CAD build for the part. Positions are in the model's coordinates, mm. Round coordinates to 2 decimals unless told otherwise and drop trailing zeros. Order: outer loops, then holes, each group sorted by start corner. A loop starts at its lowest first (then second) coordinate and runs counter-clockwise, first axis right, second up. Notation, with made-up numbers: M 36,78 L 46,78 A14 ccw 46,84 Z; hole C 84.5,38 d9. An arc over 180 degrees is marked long. Answer as CSV lines item,"result". Start each with the question number.
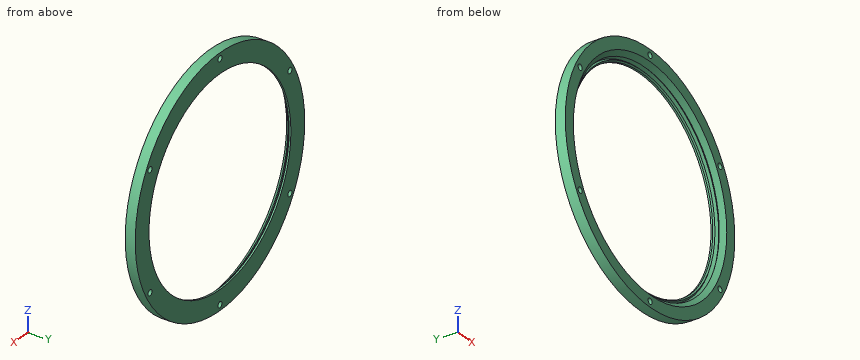
Autodesk Inventor part; units mm, degrees
ref_plane "YZ Plane" through (0, 0, 0) normal (1, 0, 0) x (0, 1, 0)
ref_plane "XZ Plane" through (0, 0, 0) normal (0, 1, 0) x (-1, 0, 0)
ref_plane "XY Plane" through (0, 0, 0) normal (0, 0, 1) x (1, 0, 0)
sketch "Sketch1" plane through (0, 0, 0) normal (0, 0, 1) x (1, 0, 0)
  line L0 (0, -12.446) -> (0, 12.446)
  line L1 (-129.54, 0) -> (21.59, 0) construction
  line L2 (-107.95, 8.89) -> (-107.95, 0)
  line L3 (-107.95, 8.89) -> (-90.3815, 8.89)
  line L4 (-90.3815, 8.89) -> (-90.3815, 7.3025)
  line L5 (-90.3815, 7.3025) -> (-91.504, 6.18)
  line L6 (-91.504, 6.18) -> (-92.9409, 7.6168)
  line L7 (-92.9409, 7.6168) -> (-95.186, 5.3717)
  line L8 (-95.186, 5.3717) -> (-93.7491, 3.9349)
  line L9 (-93.7491, 3.9349) -> (-97.684, 0)
  line L10 (-97.176, 0) -> (-88.9855, 8.1905) construction
  line L11 (-94.0634, 6.4943) -> (-92.3726, 4.8034) construction
  circle A0 centre (-93.218, 5.6489) radius 1.3081 construction
  line L12 (-107.95, -8.89) -> (-90.3815, -8.89) construction
  line L13 (-90.3815, -8.89) -> (-90.3815, -7.3025) construction
  line L14 (-90.3815, -7.3025) -> (-91.504, -6.18) construction
  line L15 (-91.504, -6.18) -> (-92.9409, -7.6168) construction
  line L16 (-92.9409, -7.6168) -> (-95.186, -5.3717) construction
  line L17 (-95.186, -5.3717) -> (-93.7491, -3.9349) construction
  line L18 (-93.7491, -3.9349) -> (-97.684, 0) construction
  line L19 (-107.95, 0) -> (-97.684, 0)
  line L20 (-107.95, 0) -> (-107.95, -8.89) construction
  point P0 (0, 0)
  dimension "d24" = 1.5875
  dimension "d25" = 2.032
  dimension "d26" = 45
  dimension "d27" = 0.508
  dimension "d28" = 3.175
  dimension "d29" = 2.6162
  dimension "d30" = 186.436
  dimension "d31" = 215.9
  dimension "d32" = 17.78
  dimension "d33" = 1.5875
revolve "Revolution1" add sketch "Sketch1" angle 360 about axis through (0, -10, 0) along (0, 1, 0)
sketch "Sketch2" plane through (0, 8.89, 0) normal (0, 1, 0) x (1, 0, 0)
  point P0 (0, 0)
  point P1 (0, 102.87)
  point P2 (-89.088, 51.435)
  point P3 (-89.088, -51.435)
  point P4 (0, -102.87)
  point P5 (89.088, -51.435)
  point P6 (89.088, 51.435)
  dimension "d36" = 102.87
  dimension "d39" = 360
hole "Hole1" at (0, 8.89, -102.87) at (-89.088, 8.89, -51.435) at (-89.088, 8.89, 51.435) at (0, 8.89, 102.87) at (89.088, 8.89, 51.435) at (89.088, 8.89, -51.435) direction (0, -1, 0) diameter 5.1054 end through all
properties part number "3DPRINT,OUTER-V" material "Nylon 6/6"
Q1. Band-saw the part on B-B, the plane z = 0. Write the cut outline in (x, y).
Q2. Drop flat-ended pins along their axis: P1, Ø1, axis at y = 5.5, z = -40.5, coming from the +X side; P2, Ø1, axis at y = 5, z = 79, coming from the -X side; P3, Ø6, axis at x = -89.088, z = 51.435, coming from the -Y side; P4, Ø2, axis at x = 19.5, y = 6.5, coming from the +Z side. Give the stop position or say it passes through.
Q3. Band-saw the part on D-D, the plane z = -102.87. Write the cut outline in (x, y).
Q4. Probe line 1 along Z through (x, y) = (2, 5); line 2 along Z through (x, y) = (6.5, 6.5); line 3 along X through (y, z) = (6.75, -71). List the from-to ranges inside material, lowest first. Write a range as from..to.
Q5. Band-saw the part on A-A, the plane x = 0. Write the cut outline in (y, z), then the cut area to 3 significant figures.
Q6. Band-saw the part on C-C, the plane y = 2.5. Write the cut outline in (x, z) (3 decimals).
Answer:
1,outline,"M -107.95,0 L -97.68,0 L -93.75,3.93 L -95.19,5.37 L -92.94,7.62 L -91.5,6.18 L -90.38,7.3 L -90.38,8.89 L -107.95,8.89 Z; M 90.38,7.3 L 91.5,6.18 L 92.94,7.62 L 95.19,5.37 L 93.75,3.93 L 97.68,0 L 107.95,0 L 107.95,8.89 L 90.38,8.89 Z"
2,P1,"stops at x = 100.27"
2,P2,"stops at x = -74.1"
2,P3,"stops at y = 0"
2,P4,"stops at z = 106.35"
3,outline,"M -32.73,0 L -2.55,0 L -2.55,8.89 L -32.73,8.89 Z; M 2.55,0 L 32.73,0 L 32.73,8.89 L 2.55,8.89 Z"
4,line 1,"z = -107.93..-104.46, -101.28..-94.79, 94.79..101.28, 104.46..107.93"
4,line 2,"z = -107.75..-93.83, -91.59..-90.95, 90.95..91.59, 93.83..107.75"
4,line 3,"x = -81.32..-61.31, -58.62..-56.82, 56.82..58.62, 61.31..81.32"
5,outline,"M 0,-107.95 L 8.89,-107.95 L 8.89,-105.42 L 0,-105.42 Z; M 0,-100.32 L 8.89,-100.32 L 8.89,-90.38 L 7.3,-90.38 L 6.18,-91.5 L 7.62,-92.94 L 5.37,-95.19 L 3.93,-93.75 L 0,-97.68 Z; M 0,97.68 L 3.93,93.75 L 5.37,95.19 L 7.62,92.94 L 6.18,91.5 L 7.3,90.38 L 8.89,90.38 L 8.89,100.32 L 0,100.32 Z; M 0,105.42 L 8.89,105.42 L 8.89,107.95 L 0,107.95 Z"
5,area,"155 mm^2"
6,outline,"C 0,0 d215.9; hole C 0,0 d190.368; hole C -89.088,-51.435 d5.105; hole C -89.088,51.435 d5.105; hole C 0,-102.87 d5.105; hole C 0,102.87 d5.105; hole C 89.088,-51.435 d5.105; hole C 89.088,51.435 d5.105"
